For this review, take the finished solid that the model builds, in its own axes (mm). Face numbers are marked on the shaded views. A direction names the side the tool comes from. Coordinates: 2 decimals unless noted, no trailing zeros. Write each loop counter-clockwise with the first axis right and the second up, starting at its lowest first coordinate (ties: lowest second). Pieces come first, ordered by that corner, then holes. Notation, with made-up numbers: (25.5, -3.75) -> (43.5, -3.75) arc R27 ccw to (43.5, 24.25) -> close; hole circle Ø1 at (78.5, -17). An arc over 180 degrees is marked (long way). One line per item, written item: value. Start each with the question number.
1) For probe 1 along X at (y, z) = (-3.5, 110.5) (3 decimals); probe 2 along Y at (x, z) = (4.5, 40) (3 decimals); probe 3 along X at (y, z) = (-8, 22), list the stretches that pass through material, from the lowest coordinate up. Write a range as from..to.
2) Add section C-C (z = 11). State the section outline as (x, y) points (3 decimals).
3) Mouldability with a two-part tool opening along Z and no side actions: class the marked faces 4, 5 and 6 as released by +Z, released by -Z, zero draft, split by the parting line, or undercut.
4) Add section A-A (x = 0). State the section outline as (y, z) points (3 decimals), and give its area (3 significant figures).
5) Add section D-D (z = 110.5). State the section outline as (x, y) points (3 decimals), and give its area (3 significant figures).
6) Add section B-B (y = 2). State the section outline as (x, z) points (1 decimal), and give its area (3 significant figures).
7) Machinability: for the marked faces 1, 2 and 3, which of the approach directions +Z, -Z, +X, -X, +Y, -Y give a long, thin tool a straight path to every point of the face, cutting with its end or side? Answer none if there is none.
8) For pin 1 Ø2.5 at (y, z) = (7.5, 36.5) entering from +X (3 decimals); pin 2 Ø1.5 at (x, y) = (4, -19) entering from -Z; pin 3 Ø3 at (x, z) = (-7.5, 34) entering from -Y; pin 4 Ø2 at (x, y) = (23, 6) entering from +Z, all flat-tipped, find the tip position at first contact; note any pin that passes through.
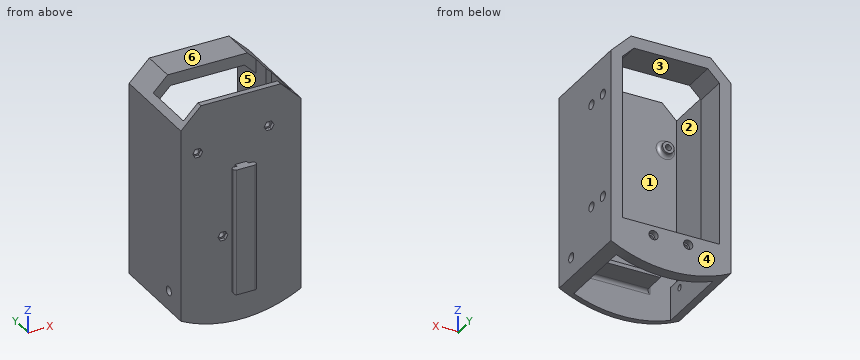
from build123d import *

# Parameters (mm, degrees)
SKETCH1_W                 = 66.04
SKETCH1_H                 = 52.07
SKETCH1_W_2               = 53.34
SKETCH1_H_2               = 42.545
BOSS_EXTRUDE1_DEPTH       = 152.4
SKETCH3_W                 = 53.34
SKETCH3_H                 = 129.7432
CUT_EXTRUDE2_DEPTH        = 48.895
BOSS_EXTRUDE3_DEPTH       = 48.895
SKETCH6_W                 = 177.8
SKETCH6_H                 = 203.2
CUT_EXTRUDE3_DEPTH        = 165.400016119
F_4_CLEARANCE_HOLE3_D     = 3.2639
F_4_CLEARANCE_HOLE3_DEPTH = 6.35
SKETCH12_R                = 2.54
CUT_EXTRUDE5_DEPTH        = 3.175
SKETCH15_R                = 2.54
CUT_EXTRUDE6_DEPTH        = 3.175
CUT_EXTRUDE9_DEPTH        = 101.854
SKETCH18_W                = 29.718
SKETCH18_H                = 4.88696
SD_CARD_HOLDER_DEPTH      = 13.9954
SKETCH19_W                = 24.3332
SKETCH19_H                = 5.6388
CUT_EXTRUDE10_DEPTH       = 2.794
SKETCH20_R                = 3.175
MOUNT_POST_DEPTH          = 3
F_4_CLEARANCE_HOLE1_D     = 3.2639
CUT_EXTRUDE11_DEPTH       = 1.905
F_4_CLEARANCE_HOLE2_D     = 3.2639
F_4_CLEARANCE_HOLE2_DEPTH = 6.35
SKETCH27_R                = 2.54
CUT_EXTRUDE13_DEPTH       = 3.175
FILLET1_R                 = 1.905
FILLET2_R                 = 1.905
CUT_EXTRUDE15_START       = -52.07
CUT_EXTRUDE15_DEPTH       = 52.07
BOSS_EXTRUDE8_DEPTH       = 107.95
FILLET3_R                 = 1.27
SKETCH32_W                = 38.1
SKETCH32_H                = 6.35
CUT_EXTRUDE16_DEPTH       = 146.211577855


with BuildPart() as part:
    # Sketch1 → Boss-Extrude1 (new body)
    with BuildSketch(Plane.XY):
        Rectangle(SKETCH1_W, SKETCH1_H)
        with Locations((0, -1.5875)):
            Rectangle(SKETCH1_W_2, SKETCH1_H_2, mode=Mode.SUBTRACT)
    extrude(amount=BOSS_EXTRUDE1_DEPTH)

    # Sketch3 → Cut-Extrude2 (cut)
    with BuildSketch(Plane(origin=(0, 26.035, 0), x_dir=(1, 0, 0), z_dir=(0, 1, 0))):
        with Locations((0, -87.5284)):
            Rectangle(SKETCH3_W, SKETCH3_H)
    extrude(amount=-CUT_EXTRUDE2_DEPTH, mode=Mode.SUBTRACT)

    # Sketch5 → Boss-Extrude3 (add)
    with BuildSketch(Plane(origin=(0, 26.035, 0), x_dir=(1, 0, 0), z_dir=(0, 1, 0))):
        Polygon((20.32, -119.1768), (26.67, -119.1768), (26.67, -112.8268), align=None)
        Polygon((-26.67, -119.1768), (-20.32, -119.1768), (-26.67, -112.8268), align=None)
        Polygon((0, -152.4), (0, -119.1768), (-20.32, -119.1768), (-26.67, -119.1768), (-26.67, -152.4), align=None)
        Polygon((26.67, -152.4), (26.67, -119.1768), (20.32, -119.1768), (0, -119.1768), (0, -152.4), align=None)
    extrude(amount=-BOSS_EXTRUDE3_DEPTH)

    # Sketch6 → Cut-Extrude3 (cut, through all)
    with BuildSketch(Plane(origin=(0, 26.035, 0), x_dir=(1, 0, 0), z_dir=(0, 1, 0))):
        with Locations((2.791033984, -70.453804893)):
            Rectangle(SKETCH6_W, SKETCH6_H)
        with BuildLine():
            Line((44.5826875, -125.5268), (-44.5826875, -125.5268))
            ThreePointArc((-44.5826875, -125.5268), (-69.844182534, -70.853519983), (-43.18, -16.850445544))
            Line((-43.18, -16.850445544), (-44.357636364, -15.353048604))
            ThreePointArc((-44.357636364, -15.353048604), (0, 0), (44.357636364, -15.353048604))
            Line((44.357636364, -15.353048604), (43.18, -16.850445544))
            ThreePointArc((43.18, -16.850445544), (69.844182534, -70.853519983), (44.5826875, -125.5268))
        make_face(mode=Mode.SUBTRACT)
    extrude(amount=-CUT_EXTRUDE3_DEPTH, mode=Mode.SUBTRACT)

    # #4 Clearance Hole3
    with Locations(Plane(origin=(0, 26.035, 0), x_dir=(1, 0, 0), z_dir=(0, 1, 0))):
        with Locations((-9.525, -17.5768), (9.525, -17.5768)):
            Hole(F_4_CLEARANCE_HOLE3_D / 2, depth=F_4_CLEARANCE_HOLE3_DEPTH)

    # Sketch12 → Cut-Extrude5 (cut)
    with BuildSketch(Plane(origin=(0, 26.035, 0), x_dir=(1, 0, 0), z_dir=(0, 1, 0))):
        with Locations(Location((-9.525, -17.5768, 0), (0, 0, 180))):
            Circle(SKETCH12_R)
        with Locations(Location((9.525, -17.5768, 0), (0, 0, 180))):
            Circle(SKETCH12_R)
    extrude(amount=-CUT_EXTRUDE5_DEPTH, mode=Mode.SUBTRACT)

    # Sketch13 → #4 Clearance Hole4 (revolve, cut)
    with BuildSketch(Plane(origin=(-26.67, -13.9065, 18.8468), x_dir=(0, 0, -1), z_dir=(0, 1, 0))):
        Polygon((0, 0), (0, 13.680574487), (1.63195, 12.7), (1.63195, 0), align=None)
    f_4_clearance_hole4 = revolve(axis=Axis((-20.32, -13.9065, 18.8468), (-1, 0, 0)), mode=Mode.SUBTRACT)

    # Sketch15 → Cut-Extrude6 (cut)
    with BuildSketch(Plane.ZY.offset(33.02)):
        with Locations((18.8468, -13.9065)):
            Circle(SKETCH15_R)
    cut_extrude6 = extrude(amount=-CUT_EXTRUDE6_DEPTH, mode=Mode.SUBTRACT)

    # Mirror1: #4 Clearance Hole4, Cut-Extrude6 across plane
    add(f_4_clearance_hole4.mirror(Plane(origin=(0, 0, 0), x_dir=(0, 0, 1), z_dir=(1, 0, 0))), mode=Mode.SUBTRACT)
    add(cut_extrude6.mirror(Plane(origin=(0, 0, 0), x_dir=(0, 0, 1), z_dir=(1, 0, 0))), mode=Mode.SUBTRACT)

    # Sketch16 → Cut-Extrude9 (cut)
    with BuildSketch(Plane(origin=(0, 0, 125.5268), x_dir=(-1, 0, 0), z_dir=(0, 0, -1))):
        Polygon((-26.67, 7.62), (29.845, 7.62), (29.845, -22.86), (-29.845, -22.86), (-29.845, -2.54), (-26.67, -2.54), align=None)
    extrude(amount=CUT_EXTRUDE9_DEPTH, mode=Mode.SUBTRACT)

    # Sketch18 → SD card holder (add)
    with BuildSketch(Plane(origin=(0, -22.86, 0), x_dir=(1, 0, 0), z_dir=(0, 1, 0))):
        with Locations((1.524, -20.65528)):
            Rectangle(SKETCH18_W, SKETCH18_H)
    extrude(amount=SD_CARD_HOLDER_DEPTH)

    # Sketch19 → Cut-Extrude10 (cut)
    with BuildSketch(Plane.XY.offset(23.09876)):
        with Locations((2.1209, -11.684)):
            Rectangle(SKETCH19_W, SKETCH19_H)
    extrude(amount=-CUT_EXTRUDE10_DEPTH, mode=Mode.SUBTRACT)

    # Sketch20 → mount post (add)
    with BuildSketch(Plane(origin=(0, -22.86, 0), x_dir=(1, 0, 0), z_dir=(0, 1, 0))):
        with Locations(Location((-9.88187, -49.20376, 0), (0, 0, 180))):
            Circle(SKETCH20_R)
        with Locations(Location((15.51813, -103.81376, 0), (0, 0, 180))):
            Circle(SKETCH20_R)
        with Locations(Location((-23.72487, -99.50846, 0), (0, 0, 180))):
            Circle(SKETCH20_R)
    extrude(amount=MOUNT_POST_DEPTH)

    # #4 Clearance Hole1 (through all)
    with Locations(Plane(origin=(0, -19.86, 0), x_dir=(1, 0, 0), z_dir=(0, 1, 0))):
        with Locations((15.51813, -103.81376), (-9.88187, -49.20376), (-23.72487, -99.50846)):
            Hole(F_4_CLEARANCE_HOLE1_D / 2)

    # Sketch23 → Cut-Extrude11 (cut)
    with BuildSketch(Plane.XZ.offset(26.035)):
        Polygon((-7.154236388, 49.20376), (-8.518053194, 51.56596), (-11.245686806, 51.56596), (-12.609503612, 49.20376), (-11.245686806, 46.84156), (-8.518053194, 46.84156), align=None)
        Polygon((18.245763612, 103.81376), (16.881946806, 106.17596), (14.154313194, 106.17596), (12.790496388, 103.81376), (14.154313194, 101.45156), (16.881946806, 101.45156), align=None)
        Polygon((-22.361053194, 97.14626), (-20.997236388, 99.50846), (-22.361053194, 101.87066), (-25.088686806, 101.87066), (-26.452503612, 99.50846), (-25.088686806, 97.14626), align=None)
    extrude(amount=-CUT_EXTRUDE11_DEPTH, mode=Mode.SUBTRACT)

    # #4 Clearance Hole2
    with Locations(Plane(origin=(33.02, 0, 0), x_dir=(0, 0, -1), z_dir=(1, 0, 0))):
        with Locations((-94.0308, 17.93875), (-94.0308, 6.50875), (-36.8808, 17.93875), (-36.8808, 6.50875)):
            Hole(F_4_CLEARANCE_HOLE2_D / 2, depth=F_4_CLEARANCE_HOLE2_DEPTH)

    # Sketch27 → Cut-Extrude13 (cut)
    with BuildSketch(Plane(origin=(33.02, 0, 0), x_dir=(0, 0, -1), z_dir=(1, 0, 0))):
        with Locations((-94.0308, 17.93875)):
            Circle(SKETCH27_R)
        with Locations((-94.0308, 6.50875)):
            Circle(SKETCH27_R)
        with Locations((-36.8808, 17.93875)):
            Circle(SKETCH27_R)
        with Locations((-36.8808, 6.50875)):
            Circle(SKETCH27_R)
    extrude(amount=-CUT_EXTRUDE13_DEPTH, mode=Mode.SUBTRACT)

    # Fillet1
    fillet1_edges = [part.edges().sort_by_distance(p)[0] for p in [
        (-13.335, -22.86, 20.65528),
        (16.383, -22.86, 20.65528),
        (1.524, -22.86, 18.2118),
    ]]
    fillet(fillet1_edges, radius=FILLET1_R)

    # Fillet2
    fillet2_edges = [part.edges().sort_by_distance(p)[0] for p in [
        (-6.70687, -22.86, 49.20376),
        (18.69313, -22.86, 103.81376),
        (-20.54987, -22.86, 99.50846),
    ]]
    fillet(fillet2_edges, radius=FILLET2_R)

    # Sketch28 → Cut-Extrude15 (cut)
    with BuildSketch(Plane(origin=(0, 26.035, 0), x_dir=(1, 0, 0), z_dir=(0, 1, 0)).offset(CUT_EXTRUDE15_START)):
        Polygon((40.411152545, -107.038724254), (0, -147.449876798), (-40.411152545, -107.038724254), (-54.779562339, -121.407134047), (0, -176.186696386), (54.779562339, -121.407134047), align=None)
    extrude(amount=CUT_EXTRUDE15_DEPTH, mode=Mode.SUBTRACT)

    # Sketch31 → Boss-Extrude8 (add)
    with BuildSketch(Plane.XY.offset(125.5268)):
        Polygon((3.175, -26.035), (-3.175, -26.035), (-3.175, -27.94), (-6.35, -27.94), (-6.35, -31.115), (6.35, -31.115), (6.35, -27.94), (3.175, -27.94), align=None)
    extrude(amount=-BOSS_EXTRUDE8_DEPTH)

    # Fillet3
    fillet3_edges = [part.edges().sort_by_distance(p)[0] for p in [
        (6.35, -29.5275, 125.5268),
        (6.35, -27.94, 71.5518),
        (6.35, -31.115, 71.5518),
        (-6.35, -29.5275, 17.5768),
        (-6.35, -31.115, 71.5518),
        (-6.35, -27.94, 71.5518),
        (6.35, -29.5275, 17.5768),
        (-6.35, -29.5275, 125.5268),
    ]]
    fillet(fillet3_edges, radius=FILLET3_R)

    # Sketch32 → Cut-Extrude16 (cut, through all)
    with BuildSketch(Plane.ZY.offset(33.02)):
        with Locations((106.4768, -29.21)):
            Rectangle(SKETCH32_W, SKETCH32_H)
    extrude(amount=-CUT_EXTRUDE16_DEPTH, mode=Mode.SUBTRACT)


solid = part.part
Numbers:
1. probe 1: -33.02..-29.845, 29.845..33.02
1. probe 2: -31.115..-27.94, -26.035..-22.86
1. probe 3: -33.02..-26.67, 26.67..33.02
2. outline: (-33.02, -26.035) -> (33.02, -26.035) -> (33.02, 26.035) -> (-33.02, 26.035) -> close; hole (-26.67, -22.86) -> (26.67, -22.86) -> (26.67, 19.685) -> (-26.67, 19.685) -> close
3. face 4: zero draft
3. face 5: undercut
3. face 6: released by +Z
4. outline: (-31.115, 17.577) -> (-26.035, 17.577) -> (-26.035, 0) -> (-22.86, 0) -> (-22.86, 16.307) arc R1.905 cw to (-20.955, 18.212) -> (-8.865, 18.212) -> (-8.865, 20.305) -> (-14.503, 20.305) -> (-14.503, 23.099) -> (-22.86, 23.099) -> (-22.86, 125.527) -> (-26.035, 125.527) -> (-26.035, 87.427) -> (-31.115, 87.427) -> close; (7.62, 119.177) -> (26.035, 119.177) -> (26.035, 125.527) -> (7.62, 125.527) -> close; (19.685, 0) -> (26.035, 0) -> (26.035, 22.657) -> (19.685, 22.657) -> close
4. area: 1,070 mm²
5. outline: (-33.02, -26.035) -> (33.02, -26.035) -> (33.02, 26.035) -> (26.67, 26.035) -> (26.67, -2.54) -> (29.845, -2.54) -> (29.845, -22.86) -> (-29.845, -22.86) -> (-29.845, 7.62) -> (-26.67, 7.62) -> (-26.67, 26.035) -> (-33.02, 26.035) -> close
5. area: 669 mm²
6. outline: (-33, 8) arc R71.8 ccw to (-26.7, 5.1) -> (-26.7, 23.7) -> (-29.8, 23.7) -> (-29.8, 117.6) -> (-33, 114.4) -> close; (26.7, 5.1) arc R71.8 ccw to (33, 8) -> (33, 114.4) -> (26.7, 120.8) -> close
6. area: 1,110 mm²
7. face 1: none
7. face 2: +Z
7. face 3: +Y
8. pin 1: x = 29.845
8. pin 2: z = 18.21
8. pin 3: y = -30.72
8. pin 4: through
